```python
from build123d import *

# Parameters (mm, degrees)
SKETCH001_W  = 95
SKETCH001_H  = 179
PAD001_DEPTH = 10
POCKET_DEPTH = 8
FILLET_R     = 3


with BuildPart() as part:
    # Sketch001 → Pad001 (new body)
    with BuildSketch(Plane.XY):
        with Locations((47.5, 89.5)):
            Rectangle(SKETCH001_W, SKETCH001_H)
    extrude(amount=PAD001_DEPTH)

    # Sketch → Pocket (cut)
    with BuildSketch(Plane.XY):
        with BuildLine():
            Line((17, 169), (78, 169))
            ThreePointArc((85, 162), (82.949747, 166.949747), (78, 169))
            Line((85, 162), (85, 17))
            ThreePointArc((78, 10), (82.949747, 12.050253), (85, 17))
            Line((78, 10), (17, 10))
            ThreePointArc((10, 17), (12.050253, 12.050253), (17, 10))
            Line((10, 17), (10, 162))
            ThreePointArc((17, 169), (12.050253, 166.949747), (10, 162))
        make_face()
    extrude(amount=POCKET_DEPTH, mode=Mode.SUBTRACT)

    # Fillet
    fillet_edges = [part.edges().sort_by_distance(p)[0] for p in [
        (10, 89.5, 8),
    ]]
    fillet(fillet_edges, radius=FILLET_R)


solid = part.part
```
For this review, take the finished solid that the model builds, in its own axes (mm). A direction names the side the tool comes from. Give positions to 0.01 mm unless a question says otherwise; leave off trailing zeros. Write each loop counter-clockwise with the first axis right and the second up, starting at its lowest first coordinate (ties: lowest second). Pieces come first, ordered by that corner, then holes.
Item 1: The part is to be moulded in two halves that separate along Y. For faces 3 (the face through (47, 0, 5)), 4 (the face through (9, 97, 0)), 5 (the face through (12, 12.1, 2.5)), 6 (the face through (47, 179, 5)), say which applies: +Y half, -Y half, draft (parallel to the pull), parting line (faces both ways), or undercut.
Item 2: Take a section at C-C (x = 25.5). Give the boundary of the cut face in (y, z).
Item 3: Machinability: for faces 1 (the face through (95, 88, 5)), 2 (the face through (47, 169, 2)), which of the approach directions +Z, -Z, +X, -X, +Y, -Y give a long, thin tool a straight path to every point of the face, cutting with its end or side? Answer none if there is none.
Item 4: Insertion check: P1, Ø6, axis at x = 25, y = 45, coming from the -Z side. The pin has a flat end and moves straight along its axis. Give the tip position at first contact, or say it passes through.
Item 5: Take a section at A-A (z = 1.5). Give the boundary of the cut face in (x, y).
Item 6: Wall thickness on probe 1 along Y at (x, z) = (51.5, 2.75); probe 2 along X at (y, z) = (37, 1.25); probe 3 along Z at (x, y) = (48.5, 95): over which ranges is each line inside the solid? List them lowest first.
Item 7: Take a section at B-B (y = 134). Give the boundary of the cut face in (x, z).
Established:
1. face 3: -Y half
1. face 4: draft
1. face 5: undercut
1. face 6: +Y half
2. outline: (0, 0) - (10, 0) - (10, 5) arc R3 cw to (13, 8) - (166, 8) arc R3 cw to (169, 5) - (169, 0) - (179, 0) - (179, 10) - (0, 10) - close
3. face 1: +Z, -Z, +X, +Y, -Y
3. face 2: -Z
4. P1: stops at z = 8
5. outline: (0, 0) - (95, 0) - (95, 179) - (0, 179) - close; hole (10, 17) arc R7 ccw to (17, 10) - (78, 10) arc R7 ccw to (85, 17) - (85, 162) arc R7 ccw to (78, 169) - (17, 169) arc R7 ccw to (10, 162) - close
6. probe 1: y = 0 to 10, 169 to 179
6. probe 2: x = 0 to 10, 85 to 95
6. probe 3: z = 8 to 10
7. outline: (0, 0) - (10, 0) - (10, 5) arc R3 cw to (13, 8) - (82, 8) arc R3 cw to (85, 5) - (85, 0) - (95, 0) - (95, 10) - (0, 10) - close
